from build123d import *

# Parameters (mm, degrees)
F0_R     = 8
F1_DEPTH = 5


with BuildPart() as f1:
    # F0 (on Top) → F1 (new body)
    with BuildSketch(Plane.XY):
        with BuildLine():
            ThreePointArc((38.8490344373, -7.4982368866), (35.8718628785, 1.471244496), (28.1221549341, 6.8802345627))
            ThreePointArc((28.1221549341, 6.8802345627), (27.2226565904, 6.5535105265), (26.3041545683, 6.2848101329))
            ThreePointArc((26.3041545683, 6.2848101329), (34.5815011117, 1.4914326892), (37.8490344373, -7.4982368866))
            ThreePointArc((37.8490344373, -7.4982368866), (35.7302878123, -14.9033579686), (30.0153461175, -20.0671111506))
            Line((30.0153461175, -20.0671111506), (26.2122119316, -22.3109136241))
            ThreePointArc((26.2122119316, -22.3109136241), (28.4028713862, -21.790282543), (30.4909167926, -20.9476011385))
            ThreePointArc((30.4909167926, -20.9476011385), (36.5892902301, -15.41567854), (38.8490344373, -7.4982368866))
        make_face()
        with BuildLine():
            ThreePointArc((11.6354406408, -16.2061715771), (11.2656060513, -15.6626309275), (10.919943616, -15.1034068738))
            Line((10.919943616, -15.1034068738), (4.6527002207, -36.1918316662))
            Line((4.6527002207, -36.1918316662), (30.4909167926, -20.9476011385))
            ThreePointArc((30.4909167926, -20.9476011385), (28.4028713862, -21.790282543), (26.2122119316, -22.3109136241))
            Line((26.2122119316, -22.3109136241), (6.3361573488, -34.0375417836))
            Line((6.3361573488, -34.0375417836), (11.6354406408, -16.2061715771))
        make_face()
        with BuildLine():
            ThreePointArc((28.1221549341, 6.8802345627), (23.1634660922, 7.4860881247), (18.2808163885, 6.4299700246))
            ThreePointArc((18.2808163885, 6.4299700246), (19.2063911412, 6.1867474035), (20.1455918313, 6.0030413071))
            ThreePointArc((20.1455918313, 6.0030413071), (23.2091706485, 6.4871331239), (26.3041545683, 6.2848101329))
            ThreePointArc((26.3041545683, 6.2848101329), (27.2226565904, 6.5535105265), (28.1221549341, 6.8802345627))
        make_face()
        with BuildLine():
            ThreePointArc((11.8690019815, -15.4202693139), (11.397115524, -15.25392267), (10.919943616, -15.1034068738))
            ThreePointArc((10.919943616, -15.1034068738), (11.2656060513, -15.6626309275), (11.6354406408, -16.2061715771))
            Line((11.6354406408, -16.2061715771), (11.8690019815, -15.4202693139))
        make_face()
        with BuildLine():
            ThreePointArc((20.1455918313, 6.0030413071), (19.2063911412, 6.1867474035), (18.2808163885, 6.4299700246))
            ThreePointArc((18.2808163885, 6.4299700246), (9.655402449, -2.646349524), (10.919943616, -15.1034068738))
            ThreePointArc((10.919943616, -15.1034068738), (11.397115524, -15.25392267), (11.8690019815, -15.4202693139))
            Line((11.8690019815, -15.4202693139), (12.0049821529, -14.9627144628))
            ThreePointArc((12.0049821529, -14.9627144628), (10.7982920028, -2.4308784123), (20.1455918313, 6.0030413071))
        make_face()
        with BuildLine():
            Line((26.5784435042, 22.7285549449), (8.4393064839, 18.6917133525))
            ThreePointArc((8.4393064839, 18.6917133525), (8.1876964566, 18.1152942206), (7.9121440123, 17.5499293192))
            Line((7.9121440123, 17.5499293192), (29.3867735594, 22.3290804795))
            Line((29.3867735594, 22.3290804795), (3.0820072992, 36.7533403216))
            ThreePointArc((3.0820072992, 36.7533403216), (4.7192641816, 35.4472223277), (6.158636429, 33.9257881863))
            Line((6.158636429, 33.9257881863), (26.5784435042, 22.7285549449))
        make_face()
        with BuildLine():
            ThreePointArc((7.9121440123, 17.5499293192), (8.1876964566, 18.1152942206), (8.4393064839, 18.6917133525))
            Line((8.4393064839, 18.6917133525), (7.7274834193, 18.5332980458))
            ThreePointArc((7.7274834193, 18.5332980458), (7.8116121335, 18.0400735592), (7.9121440123, 17.5499293192))
        make_face()
        with BuildLine():
            ThreePointArc((-14.4218573571, 12.3962462122), (-2.0581580843, 9.7870747046), (7.9121440123, 17.5499293192))
            ThreePointArc((7.9121440123, 17.5499293192), (7.8116121335, 18.0400735592), (7.7274834193, 18.5332980458))
            Line((7.7274834193, 18.5332980458), (7.2272436675, 18.421970333))
            ThreePointArc((7.2272436675, 18.421970333), (-2.7467318854, 10.6627009825), (-14.907533277, 14.0980115505))
            ThreePointArc((-14.907533277, 14.0980115505), (-14.6395764677, 13.2542976843), (-14.4218573571, 12.3962462122))
        make_face()
        with BuildLine():
            Line((2.555704028, 35.9014618202), (6.158636429, 33.9257881863))
            ThreePointArc((6.158636429, 33.9257881863), (4.7192641816, 35.4472223277), (3.0820072992, 36.7533403216))
            ThreePointArc((3.0820072992, 36.7533403216), (-13.8153698815, 36.8408290348), (-20.0726464643, 21.144475967))
            ThreePointArc((-20.0726464643, 21.144475967), (-19.3800207125, 20.593183388), (-18.7211221359, 20.0019925512))
            ThreePointArc((-18.7211221359, 20.0019925512), (-13.8112245946, 35.6176830282), (2.555704028, 35.9014618202))
        make_face()
        with BuildLine():
            ThreePointArc((-20.0726464643, 21.144475967), (-18.0308595518, 16.2642013697), (-14.4218573571, 12.3962462122))
            ThreePointArc((-14.4218573571, 12.3962462122), (-14.6395764677, 13.2542976843), (-14.907533277, 14.0980115505))
            ThreePointArc((-14.907533277, 14.0980115505), (-17.1908591544, 16.8067871532), (-18.7211221359, 20.0019925512))
            ThreePointArc((-18.7211221359, 20.0019925512), (-19.3800207125, 20.593183388), (-20.0726464643, 21.144475967))
        make_face()
        with BuildLine():
            ThreePointArc((-8.275330105, -27.9556597428), (-5.0113342557, -23.6320437442), (-3.4960276219, -18.4309698155))
            ThreePointArc((-3.4960276219, -18.4309698155), (-4.1118905803, -19.0296020384), (-4.6924818025, -19.6625013626))
            ThreePointArc((-4.6924818025, -19.6625013626), (-5.9051240284, -23.183557577), (-8.003150447, -26.2603453792))
            ThreePointArc((-8.003150447, -26.2603453792), (-8.1635176407, -27.1041048739), (-8.275330105, -27.9556597428))
        make_face()
        with BuildLine():
            ThreePointArc((-32.4289424962, -11.5476477284), (-33.0476433207, -13.5913198261), (-33.3698936049, -15.7021350969))
            ThreePointArc((-33.3698936049, -15.7021350969), (-24.9998603459, -30.3836790472), (-8.275330105, -27.9556597428))
            ThreePointArc((-8.275330105, -27.9556597428), (-8.1635176407, -27.1041048739), (-8.003150447, -26.2603453792))
            ThreePointArc((-8.003150447, -26.2603453792), (-23.9694406728, -29.7571251146), (-32.3693101655, -15.7359951816))
            Line((-32.3693101655, -15.7359951816), (-32.4289424962, -11.5476477284))
        make_face()
        with BuildLine():
            ThreePointArc((-20.1895506368, -2.0097101454), (-19.5561991387, -1.947983056), (-18.9207994891, -1.9131744502))
            Line((-18.9207994891, -1.9131744502), (-33.796980576, 14.2948246944))
            Line((-33.796980576, 14.2948246944), (-33.3698936049, -15.7021350969))
            ThreePointArc((-33.3698936049, -15.7021350969), (-33.0476433207, -13.5913198261), (-32.4289424962, -11.5476477284))
            Line((-32.4289424962, -11.5476477284), (-32.7597333746, 11.6858418158))
            Line((-32.7597333746, 11.6858418158), (-20.1895506368, -2.0097101454))
        make_face()
        with BuildLine():
            ThreePointArc((-19.6800914911, -2.5647795781), (-19.2950109131, -2.2453097311), (-18.9207994891, -1.9131744502))
            ThreePointArc((-18.9207994891, -1.9131744502), (-19.5561991387, -1.947983056), (-20.1895506368, -2.0097101454))
            Line((-20.1895506368, -2.0097101454), (-19.6800914911, -2.5647795781))
        make_face()
        with BuildLine():
            ThreePointArc((-3.4181808461, -16.9047512351), (-7.9907957387, -6.1219111722), (-18.9207994891, -1.9131744502))
            ThreePointArc((-18.9207994891, -1.9131744502), (-19.2950109131, -2.2453097311), (-19.6800914911, -2.5647795781))
            Line((-19.6800914911, -2.5647795781), (-19.340160936, -2.9351430547))
            ThreePointArc((-19.340160936, -2.9351430547), (-8.8502061716, -6.6844840845), (-4.4181808461, -16.9047512351))
            ThreePointArc((-4.4181808461, -16.9047512351), (-4.4869248616, -18.2904303809), (-4.6924818025, -19.6625013626))
            ThreePointArc((-4.6924818025, -19.6625013626), (-4.1118905803, -19.0296020384), (-3.4960276219, -18.4309698155))
            ThreePointArc((-3.4960276219, -18.4309698155), (-3.4376551817, -17.6688525497), (-3.4181808461, -16.9047512351))
        make_face()
        with BuildLine():
            ThreePointArc((18.2808163885, 6.4299700246), (11.5832094425, 10.578918544), (7.9121440123, 17.5499293192))
            ThreePointArc((7.9121440123, 17.5499293192), (-2.0581580843, 9.7870747046), (-14.4218573571, 12.3962462122))
            ThreePointArc((-14.4218573571, 12.3962462122), (-14.7542295678, 4.6387919255), (-18.9207994891, -1.9131744502))
            ThreePointArc((-18.9207994891, -1.9131744502), (-7.9907957387, -6.1219111722), (-3.4181808461, -16.9047512351))
            ThreePointArc((-3.4181808461, -16.9047512351), (-3.4376551817, -17.6688525497), (-3.4960276219, -18.4309698155))
            ThreePointArc((-3.4960276219, -18.4309698155), (3.2731601147, -14.8661881946), (10.919943616, -15.1034068738))
            ThreePointArc((10.919943616, -15.1034068738), (9.655402449, -2.646349524), (18.2808163885, 6.4299700246))
        make_face()
        Circle(F0_R, mode=Mode.SUBTRACT)
    extrude(amount=F1_DEPTH)


solid = f1.part
Verification items for the finished model (mm, model axes). A direction names the side the tool comes from. Round coordinates to 2 decimals unless told otherwise and drop trailing zeros. Loops run counter-clockwise (first coordinate to the right, second up) from the corner with the lowest first, then second, coordinate; pieces in that order, holes last. Notation, with made-up numbers: (55, 70.5) - (98, 70.5) arc R4 cw to (98, 76.5) - close; hole circle Ø11 at (-18.5, 3.5). An arc over 180 degrees is marked (long way). Use a Markdown table: item, result. Add a question column.
1. Release check for a two-part mould opening along Y. For faces 4 (the face through (-14.722, 4.744, 2.465)), 5 (the face through (-6, -7, 0)), 6 (the face through (16.42, 29.44, 2.46)) record: released by +Y, released by -Y, zero draft, split by the parting line, or undercut.
2. Access from +Z, -Z, +X, -X, +Y, -Y to the whole of each face (thin tool, end or side, straight path). Record for faces 1 (the face through (-6, -7, 5)), 2 (the face through (18.499, 19.906, 2.465)), 3 (the face through (7.83, -25.5, 2.46)).
3. Section check B-B, the plane x = 0. Record the boundary of the cut face in (y, z), plus the area to 3 significant figures.
4. Gauge pin test, flat ends, axial feed: pin 1 (1 mm diameter, centred on y = 17.5, z = 2, fed in from -X); pin 2 (3 mm diameter, centred on x = 24, y = 29, fed in from -Z); pin 3 (1 mm diameter, centred on x = 26.5, z = 3.5, fed in from -Y). Record the tip position at first contact, or that the pin passes through.
5. Section check C-C, the plane y = -24. Record the boundary of the cut face in (x, z).
6. Section check A-A, the plane y = 0. Record the boundary of the cut face in (x, z), plus the area to 3 significant figures.
7. Section check D-D, the plane x = 13. Record the boundary of the cut face in (y, z), plus the area to 3 significant figures.
8. Thickness scan on probe 1 along Y at (x, z) = (0, 3.35); probe 2 along Y at (x, z) = (23, 3.2); probe 3 along X at (y, z) = (-27, 0.75). Record the ranges inside material, lowest first. Write a range as [from, to].
Checks:
| question | item | result |
|---|---|---|
| 1 | face 4 | undercut |
| 1 | face 5 | zero draft |
| 1 | face 6 | released by +Y |
| 2 | face 1 | +Z, +X, -X, +Y, -Y |
| 2 | face 2 | +Z, -Z, +X |
| 2 | face 3 | +Z, -Z |
| 3 | outline | (-16.03, 0) - (-8, 0) - (-8, 5) - (-16.03, 5) - close; (8, 0) - (11.5, 0) - (11.5, 5) - (8, 5) - close; (37.31, 0) - (38.39, 0) - (38.39, 5) - (37.31, 5) - close |
| 3 | area | 63.1 mm^2 |
| 4 | pin 1 | stops at x = -19 |
| 4 | pin 2 | passes through |
| 4 | pin 3 | stops at y = -23.6 |
| 5 | outline | (-31.63, 0) - (-30.49, 0) - (-30.49, 5) - (-31.63, 5) - close; (-6.35, 0) - (-5.2, 0) - (-5.2, 5) - (-6.35, 5) - close; (8.28, 0) - (9.32, 0) - (9.32, 5) - (8.28, 5) - close; (23.35, 0) - (25.32, 0) - (25.32, 5) - (23.35, 5) - close |
| 6 | outline | (-33.59, 0) - (-32.59, 0) - (-32.59, 5) - (-33.59, 5) - close; (-22.03, 0) - (-20.68, 0) - (-20.68, 5) - (-22.03, 5) - close; (-17.17, 0) - (-8, 0) - (-8, 5) - (-17.17, 5) - close; (8, 0) - (12.03, 0) - (12.03, 5) - (8, 5) - close; (35.67, 0) - (36.84, 0) - (36.84, 5) - (35.67, 5) - close |
| 6 | area | 83.6 mm^2 |
| 7 | outline | (-31.27, 0) - (-30.11, 0) - (-30.11, 5) - (-31.27, 5) - close; (1.35, 0) - (9.24, 0) - (9.24, 5) - (1.35, 5) - close; (18.68, 0) - (19.71, 0) - (19.71, 5) - (18.68, 5) - close; (30.17, 0) - (31.31, 0) - (31.31, 5) - (30.17, 5) - close |
| 7 | area | 56.1 mm^2 |
| 8 | probe 1 | y = [-16.03, -8], [8, 11.5], [37.31, 38.39] |
| 8 | probe 2 | y = [-25.37, -24.21], [6.48, 7.48], [20.91, 21.93], [24.69, 25.83] |
| 8 | probe 3 | x = [-29.51, -28.12], [-8.72, -7.32], [7.38, 8.43], [18.26, 20.23] |
